CAD build for the part. Positions are in the model's coordinates, mm. Face numbers are marked on the shaded views. A direction names the side the tool comes from. Coordinates: 2 decimals unless noted, no trailing zeros. Order: outer loops, then holes, each group sorted by start corner. A loop starts at its lowest first (then second) coordinate and runs counter-clockwise, first axis right, second up.
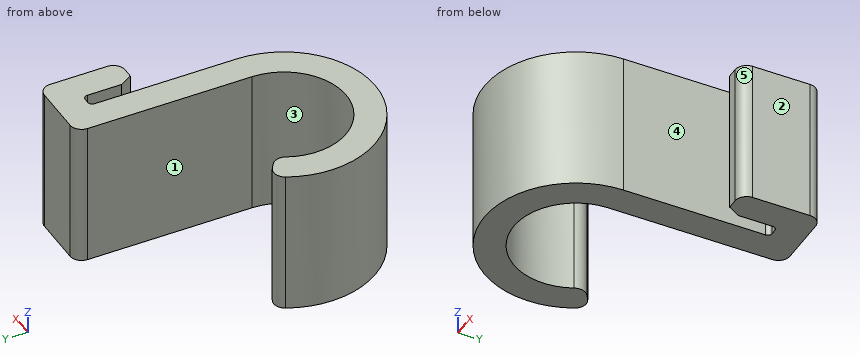
from build123d import *

# Parameters (mm, degrees)
F1_DEPTH = 25.4
F2_R     = 0.762
F3_R     = 2.032
F4_SIZE2 = 2.1997045256
F4_SIZE  = 1.27


with BuildPart() as f1:
    # F0 (on Top) → F1 (new body)
    with BuildSketch(Plane.XY):
        with BuildLine():
            ThreePointArc((10.7569, 0), (-3.2346622147, -10.2590378675), (-8.8115366252, 6.1699043682))
            Line((-8.8115366252, 6.1699043682), (-12.9728290102, 9.0836726648))
            ThreePointArc((-12.9728290102, 9.0836726648), (-4.7622476762, -15.1039199773), (15.8369, 0))
            Line((15.8369, 0), (15.8369, 25.4))
            Line((15.8369, 25.4), (18.2499, 25.4))
            Line((18.2499, 25.4), (18.2499, 16.51))
            Line((18.2499, 16.51), (23.3299, 16.51))
            Line((23.3299, 16.51), (23.3299, 30.48))
            Line((23.3299, 30.48), (10.7569, 30.48))
            Line((10.7569, 30.48), (10.7569, 0))
        make_face()
    extrude(amount=F1_DEPTH)

    # F2
    f2_edges = [f1.edges().sort_by_distance(p)[0] for p in [
        (15.8369, 25.4, 12.7),
        (18.2499, 25.4, 12.7),
    ]]
    fillet(f2_edges, radius=F2_R)

    # F3
    f3_edges = [f1.edges().sort_by_distance(p)[0] for p in [
        (23.3299, 16.51, 12.7),
        (23.3299, 30.48, 12.7),
        (10.7569, 30.48, 12.7),
        (-8.811537, 6.169904, 12.7),
        (-12.972829, 9.083673, 12.7),
    ]]
    fillet(f3_edges, radius=F3_R)

    # F4
    f4_edges = [f1.edges().sort_by_distance(p)[0] for p in [
        (18.2499, 16.51, 12.7),
    ]]
    f4_side = f1.faces().sort_by_distance((19.7739, 16.51, 12.7))[0]
    chamfer(f4_edges, length=F4_SIZE, length2=F4_SIZE2, reference=f4_side)


solid = f1.part
1) Which spindle directions (+Z, -Z, +X, -X, +Y, -Y) get a long thin tool onto all of the face, cutting with end or side? Do the marked faces 1 and 2. Say none if no direction does.
2) Drill centre lines: probe 1 along X at (y, z) = (22, 22); probe 2 along X at (y, z) = (2.5, 19.25); probe 3 along Y at (x, z) = (0, 8.5). Where is each one in solid material? Low to high.
3) Slice it at D-D (x = 0). List the corners of the cut face in (y, z).
4) Slice it at C-C (y = 9.5). List the corners of the cut face in (x, z).
5) Pin check, flat tips, straight feed: P1, Ø0.9, axis at x = 21, z = 7, coming from the -Y side; P2, Ø2, axis at y = 8.5, z = 7, coming from the +X side; P3, Ø12.5, axis at y = 17.5, z = 12.5, coming from the -X side. Stop position of each tip, or through.
6) Two-plate mould, pull along Y, no slides. Class the marked faces 3, 4 and 5: released by +Y, released by -Y, zero draft, split by the parting line, or undercut.
7) Slice it at B-B (z = 22). List the corners of the cut face in (x, y), plus the area to 3 significant figures.
8) Slice it at A-A (y = -1). List the corners of the cut face in (x, z), plus the area to 3 significant figures.
Worked out:
1. face 1: +Z, -Z, +Y
1. face 2: +Z, -Z, +X, +Y, -Y
2. probe 1: x = 10.76 to 15.84, 18.25 to 23.33
2. probe 2: x = -15.64 to -10.46, 10.76 to 15.84
2. probe 3: y = -15.84 to -10.76
3. outline: (-15.84, 0) - (-10.76, 0) - (-10.76, 25.4) - (-15.84, 25.4) - close
4. outline: (10.76, 0) - (15.84, 0) - (15.84, 25.4) - (10.76, 25.4) - close
5. P1: stops at y = 16.51
5. P2: stops at x = 15.84
5. P3: stops at x = 10.76
6. face 3: undercut
6. face 4: zero draft
6. face 5: released by -Y
7. outline: (-14.17, 7.08) arc R15.84 ccw (long way) to (15.84, 0) - (15.84, 24.64) arc R0.76 cw to (16.6, 25.4) - (17.49, 25.4) arc R0.76 cw to (18.25, 24.64) - (18.25, 18.71) - (19.52, 16.51) - (21.3, 16.51) arc R2.03 ccw to (23.33, 18.54) - (23.33, 28.45) arc R2.03 ccw to (21.3, 30.48) - (12.79, 30.48) arc R2.03 ccw to (10.76, 28.45) - (10.76, 0) arc R10.76 cw (long way) to (-9.68, 4.69) arc R2.03 ccw to (-10.34, 7.24) - (-11.19, 7.83) arc R2.03 ccw to start
7. area: 486 mm2
8. outline: (-15.81, 0) - (-10.71, 0) - (-10.71, 25.4) - (-15.81, 25.4) - close; (10.71, 0) - (15.81, 0) - (15.81, 25.4) - (10.71, 25.4) - close
8. area: 259 mm2
